Autodesk Inventor part; units mm, degrees
ref_plane "YZ Plane" through (0, 0, 0) normal (1, 0, 0) x (0, 1, 0)
ref_plane "XZ Plane" through (0, 0, 0) normal (0, 1, 0) x (-1, 0, 0)
ref_plane "XY Plane" through (0, 0, 0) normal (0, 0, 1) x (1, 0, 0)
sketch "スケッチ1" plane through (0, 0, 0) normal (0, 1, 0) x (-1, 0, 0)
  circle A0 centre (0, 0) radius 15
  dimension "d0" = 30
extrude "押し出し1" add sketch "スケッチ1" along normal blind 5
sketch "スケッチ2" plane through (0, 5, 0) normal (0, 1, 0) x (1, 0, 0)
  circle A0 centre (0, 0) radius 12
  point P0 (-12, 0)
  point P1 (-6, -10.3923)
  point P2 (6, -10.3923)
  point P3 (12, 0)
  point P4 (6, 10.3923)
  point P5 (-6, 10.3923)
  dimension "d3" = 24
  dimension "d6" = 360
hole "穴1" at (-12, 5, 0) at (-6, 5, 10.3923) at (6, 5, 10.3923) at (12, 5, 0) at (6, 5, -10.3923) at (-6, 5, -10.3923) direction (0, -1, 0) diameter 3.2 end through all
properties part number "baseplate_forR2" material "アルミニウム 6061"
Read the model definition and answer for the solid it produces. Units are mm, in the model's axes. Coordinates: 2 decimals unless noted, no trailing zeros. Order: outer loops, then holes, each group sorted by start corner. A loop starts at its lowest first (then second) coordinate and runs counter-clockwise, first axis right, second up. Notation, with made-up numbers: M 89,66 L 125,66 A16 cw 125,88 Z; hole C -31,55.5 d3. An arc over 180 degrees is marked long. Put each result on its own line as item: value. Start each with the question number.
Item 1: Section D-D, the plane x = -6 is taken. Determine the outline of the cut face in (y, z), plus the area to 3 significant figures.
Item 2: Given pin 1 Ø3 at (x, y) = (1, 2) entering from -Z; pin 2 Ø3 at (x, z) = (12, 0) entering from -Y, each flat-ended and moving along its own axis, determine where each tip first touches the part or whether it passes through.
Item 3: Consider probe 1 along Z at (x, y) = (-6, 2.6); probe 2 along X at (y, z) = (3.65, -10.25); probe 3 along X at (y, z) = (4.25, -0.75). Determine where each line is inside the solid, lowest interval first. Write a range as [from, to].
Item 4: Section C-C, the plane y = 1.6 is taken. Determine the outline of the cut face in (x, z), plus the area to 3 significant figures.
Item 5: The mould has two halves that part along Z. Classify faces 1 (the face through (14.985, 2.465, -0.66)), 2 (the face through (0, 0, 0)), 3 (the face through (-4.438, 2.465, 10.045)): +Z half, -Z half, draft (parallel to the pull), parting line (faces both ways), or undercut.
Item 6: Section A-A, the plane z = 0 is taken. Determine the outline of the cut face in (x, y), plus the area to 3 significant figures.
Item 7: Section B-B, the plane x = -12 is taken. Determine the outline of the cut face in (y, z).
Computed:
1. outline: M 0,-13.75 L 5,-13.75 L 5,-11.99 L 0,-11.99 Z; M 0,-8.79 L 5,-8.79 L 5,8.79 L 0,8.79 Z; M 0,11.99 L 5,11.99 L 5,13.75 L 0,13.75 Z
1. area: 105 mm2
2. pin 1: stops at z = -15
2. pin 2: passes through
3. probe 1: z = [-13.75, -11.99], [-8.79, 8.79], [11.99, 13.75]
3. probe 2: x = [-10.95, -7.59], [-4.41, 4.41], [7.59, 10.95]
3. probe 3: x = [-14.98, -13.41], [-10.59, 10.59], [13.41, 14.98]
4. outline: C 0,0 d30; hole C -12,0 d3.2; hole C -6,-10.39 d3.2; hole C -6,10.39 d3.2; hole C 6,-10.39 d3.2; hole C 6,10.39 d3.2; hole C 12,0 d3.2
4. area: 659 mm2
5. face 1: parting line
5. face 2: draft
5. face 3: undercut
6. outline: M -15,0 L -13.6,0 L -13.6,5 L -15,5 Z; M -10.4,0 L 10.4,0 L 10.4,5 L -10.4,5 Z; M 13.6,0 L 15,0 L 15,5 L 13.6,5 Z
6. area: 118 mm2
7. outline: M 0,-9 L 5,-9 L 5,-1.6 L 0,-1.6 Z; M 0,1.6 L 5,1.6 L 5,9 L 0,9 Z
